Geometry: see drawing. Coordinates: mm, zero at the bounding-box minimum. A direction names the side the tool comes from. Give positions to 0.01 mm unless a question says otherwise; leave off trailing zeros. Order: outer loops, then holes, each group sorted by start corner. A loop starts at its lowest first (then second) coordinate and runs counter-clockwise, first axis right, second up. Notation, with made-up numbers: (-10, 18) - (3, 18) arc R25 ccw to (3, 37) - close; hole circle Ø6 at (78, -28.75). An arc over 180 degrees is marked (long way). Write item = value, one per line. Start each with the question number.
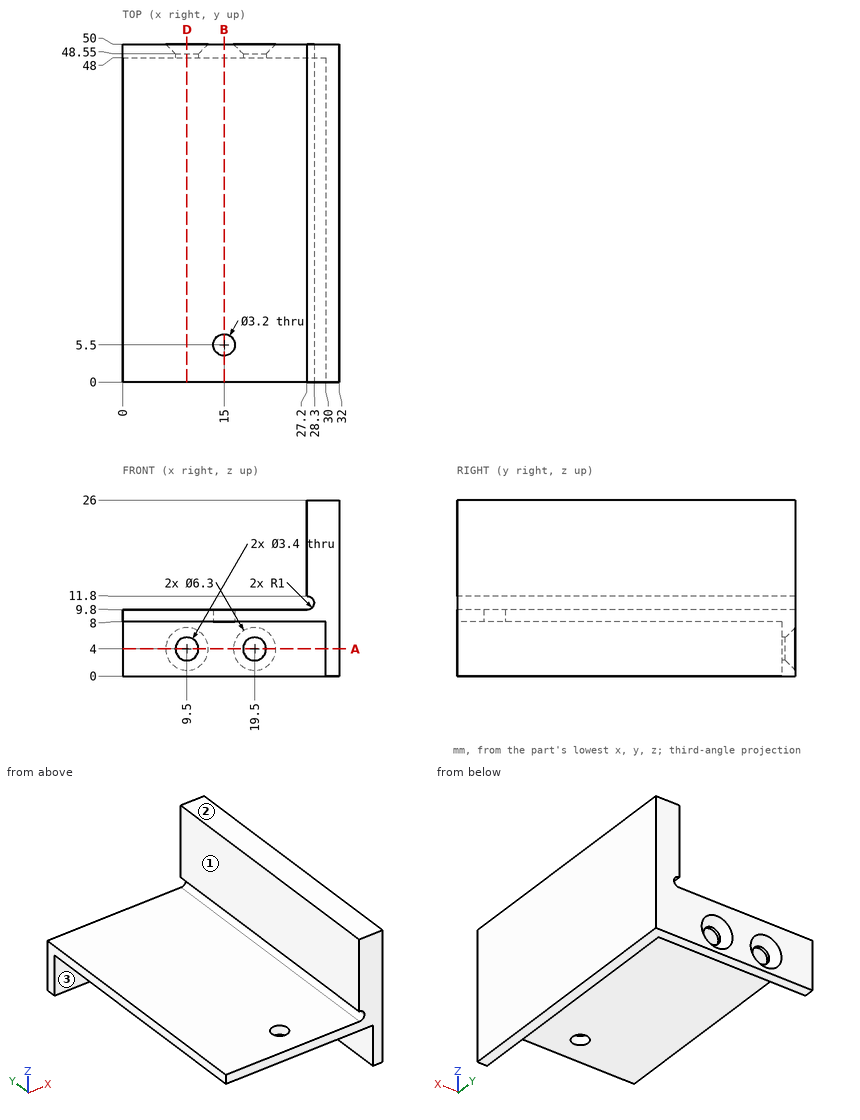
Q1. Section D-D, the plane x = 9.5. Return the cut outline in (y, z).
Q2. Section B-B, the plane x = 15. Return the cut outline in (y, z), then the cut area to 3 significant figures.
Q3. Contact query for flat-ended pins moving along their axis: pin 1 (2 mm diameter, centred on x = 19.5, z = 4, fed in from +Y); pin 2 (5 mm diameter, centred on x = 15, y = 5.5, fed in from -Z); pin 3 (1 mm diameter, centred on x = 13.5, y = 18, fed in from +Z); pin 4 (2.5 mm diameter, centred on x = 15.5, z = 6, fed in from -Y). Output: stop coordinate, or through.
Q4. Material intervals for line 1 along X through (y, z) = (48.1, 4); line 2 along Z through (x, y) = (9.5, 48.15); line 3 along Y through (x, z) = (15, 8.45), sorted ascending. Write a range as from..to.
Q5. Section A-A, the plane z = 4. Return the cut outline in (x, y).
Q6. Set-up query: the marked faces 1, 2 and 3. Return all of +Z, -Z, +X, -X, +Y, -Y with unobstructed straight access to the full face (end or side cutting, diameter ignored); none if empty.
The answers:
q1.outline = (0, 8) - (48, 8) - (48, 5.7) - (48.55, 5.7) - (50, 7.15) - (50, 9.8) - (0, 9.8) - close; (48, 0) - (50, 0) - (50, 0.85) - (48.55, 2.3) - (48, 2.3) - close
q2.outline = (0, 8) - (3.9, 8) - (3.9, 9.8) - (0, 9.8) - close; (7.1, 8) - (48, 8) - (48, 0) - (50, 0) - (50, 9.8) - (7.1, 9.8) - close
q2.area = 100 mm²
q3.pin_1 = through
q3.pin_2 = 8
q3.pin_3 = 9.8
q3.pin_4 = 48
q4.line_1 = 0..7.8, 11.2..17.8, 21.2..32
q4.line_2 = 0..2.3, 5.7..9.8
q4.line_3 = 0..3.9, 7.1..50
q5.outline = (0, 48) - (7.8, 48) - (7.8, 48.55) - (6.35, 50) - (0, 50) - close; (11.2, 48) - (17.8, 48) - (17.8, 48.55) - (16.35, 50) - (12.65, 50) - (11.2, 48.55) - close; (21.2, 48) - (30, 48) - (30, 0) - (32, 0) - (32, 50) - (22.65, 50) - (21.2, 48.55) - close
q6.face_1 = +Z, -X, +Y, -Y
q6.face_2 = +Z, +X, -X, +Y, -Y
q6.face_3 = -Z, -X, -Y
